from build123d import *

# Parameters (mm, degrees)
F1_DEPTH = 28
F2_R     = 3.15
F3_DEPTH = 40.001
F4_W     = 13
F4_H     = 17
F5_DEPTH = 32.001
F7_DEPTH = 44.4873


with BuildPart() as f1:
    # F0 (on Top) → F1 (new body)
    with BuildSketch(Plane.XY):
        with BuildLine():
            Line((16, 20), (-16, 20))
            Line((-16, 20), (-16, 16))
            Line((-16, 16), (-14, 16))
            Line((-14, 16), (5.885721, 16))
            ThreePointArc((5.885721, 16), (11.458172, 0.155277), (6.863122, -16))
            Line((6.863122, -16), (-14, -16))
            Line((-14, -16), (-16, -16))
            Line((-16, -16), (-16, -20))
            Line((-16, -20), (6.863122, -20))
            Line((6.863122, -20), (16, -24.4863))
            Line((16, -24.4863), (44, -24.4863))
            Line((44, -24.4863), (44, -20))
            Line((44, -20), (44, -13.228022))
            Line((44, -13.228022), (16, -13.228022))
            Line((16, -13.228022), (16, -10))
            Line((16, -10), (16, 20))
        make_face()
    extrude(amount=F1_DEPTH)

    # F2 (on face) → F3 (cut, through all)
    with BuildSketch(Plane.XZ.offset(20)):
        with Locations((-4.1, 14)):
            Circle(F2_R)
    extrude(amount=-F3_DEPTH, mode=Mode.SUBTRACT)

    # F4 (on face) → F5 (cut, through all)
    with BuildSketch(Plane.YZ.offset(16)):
        with Locations((2.2, 13.9)):
            Rectangle(F4_W, F4_H)
    extrude(amount=-F5_DEPTH, mode=Mode.SUBTRACT)

    # F6 (on face) → F7 (cut, through all)
    with BuildSketch(Plane.XZ.offset(24.4863)):
        with BuildLine():
            ThreePointArc((34.555264, 28), (40.804386, 23.424462), (44, 16.369312))
            Line((44, 16.369312), (44, 28))
            Line((44, 28), (34.555264, 28))
        make_face()
        with BuildLine():
            ThreePointArc((44, 11.252501), (41.099959, 4.573225), (35.433516, 0))
            Line((35.433516, 0), (44, 0))
            Line((44, 0), (44, 11.252501))
        make_face()
    extrude(amount=-F7_DEPTH, mode=Mode.SUBTRACT)


solid = f1.part
Geometry: final body of the model. Coordinates: model frame, mm. A direction names the side the tool comes from. Round coordinates to 2 decimals unless told otherwise and drop trailing zeros. Loops run counter-clockwise (first coordinate to the right, second up) from the corner with the lowest first, then second, coordinate; pieces in that order, holes last. Notation, with made-up numbers: M 44,33.5 L 78,33.5 A27 cw 78,54.5 Z; hole C 69.25,-1 d11. An arc over 180 degrees is marked long. Put each result on its own line as item: value. Start each with the question number.
(1) Section query D-D (z = 21.25). Return loops of the section in (x, y), then the cut area to 3 significant figures.
(2) Contact query for flat-ended pins moving along their axis: pin 1 Ø2 at (y, z) = (7.5, 4.5) entering from -X; pin 2 Ø10 at (x, z) = (-4.1, 14) entering from -Y; pin 3 Ø3 at (x, z) = (26, 25) entering from +Y. Output: stop coordinate, or through.
(3) Set-up query: faces 4 (the face through (44, -19, 14)), 5 (the face through (14, 2, 5.4)), 6 (the face through (-4.7, -20, 10.7)), 7 (the face through (13, -7, 28)), 8 (the face through (16, 11, 14)). Return all of +Z, -Z, +X, -X, +Y, -Y with unobstructed straight access to the full face (end or side cutting, diameter ignored); none if empty.
(4) Draft query along Z for faces 1 (the face through (13, 8.7, 14)), 2 (the face through (-4.4, -16, 10.7)), 3 (the face through (13, -7, 0)). Return one class per face: +Z half, -Z half, draft (parallel to the pull), parting line (faces both ways), or undercut.
(5) Section query A-A (x = -4.1). Return loops of the section in (y, z).
(6) Section query C-C (y = 1). Return loops of the section in (x, z), then the cut area to 3 significant figures.
(7) Material intervals for line 1 along Z through (x, y) = (-4.1, -17.55); line 2 along Y through (x, z) = (-2, 19.25); line 3 along Z through (x, y) = (15.5, -2.5), sorted ascending. Write a range as [from, to].
(8) Section query B-B (z = 14). Return loops of the section in (x, y).
Findings below:
1. outline: M -16,-20 L 6.86,-20 L 16,-24.49 L 42.28,-24.49 L 42.28,-13.23 L 16,-13.23 L 16,-4.3 L 11.24,-4.3 A27.73 cw 6.86,-16 L -16,-16 Z; M -16,16 L 5.89,16 A27.73 cw 9.83,8.7 L 16,8.7 L 16,20 L -16,20 Z
1. area: 705 mm2
2. pin 1: stops at x = 9.9
2. pin 2: stops at y = -20
2. pin 3: stops at y = -13.23
3. face 4: +Z, -Z, +X, +Y, -Y
3. face 5: +X, -X
3. face 6: +Z, -Z, -X, -Y
3. face 7: +Z, +X, -X, +Y, -Y
3. face 8: +Z, -Z, +X, +Y
4. face 1: undercut
4. face 2: draft
4. face 3: -Z half
5. outline: M -20,0 L -16,0 L -16,10.85 L -20,10.85 Z; M -20,17.15 L -16,17.15 L -16,28 L -20,28 Z; M 16,0 L 20,0 L 20,10.85 L 16,10.85 Z; M 16,17.15 L 20,17.15 L 20,28 L 16,28 Z
6. outline: M 11.42,0 L 16,0 L 16,5.4 L 11.42,5.4 Z; M 11.42,22.4 L 16,22.4 L 16,28 L 11.42,28 Z
6. area: 50.4 mm2
7. line 1: z = [0, 10.85], [17.15, 28]
7. line 2: y = [-20, -16], [16, 20]
7. line 3: z = [0, 5.4], [22.4, 28]
8. outline: M -16,-20 L -7.25,-20 L -7.25,-16 L -16,-16 Z; M -16,16 L -7.25,16 L -7.25,20 L -16,20 Z; M -0.95,-20 L 6.86,-20 L 16,-24.49 L 44,-24.49 L 44,-13.23 L 16,-13.23 L 16,-4.3 L 11.24,-4.3 A27.73 cw 6.86,-16 L -0.95,-16 Z; M -0.95,16 L 5.89,16 A27.73 cw 9.83,8.7 L 16,8.7 L 16,20 L -0.95,20 Z
